Work out the finished part from the listing and answer in its coordinate system (mm). Coordinates: 2 decimals unless noted, no trailing zeros. Loops run counter-clockwise (first coordinate to the right, second up) from the corner with the lowest first, then second, coordinate; pieces in that order, holes last. Notation, with made-up numbers: (13, 13.25) -> (38, 13.25) arc R20 ccw to (38, 26.25) -> close; hole circle Ø7 at (71.5, 34). An arc over 180 degrees is marked (long way). Use a Markdown table: item, result.
from build123d import *

# Parameters (mm, degrees)
SKETCH1_R           = 30
SKETCH1_R_2         = 1.5
BOSS_EXTRUDE1_DEPTH = 8
SKETCH2_R           = 23.65
SKETCH2_R_2         = 7.62
CUT_EXTRUDE1_DEPTH  = 8
BOSS_EXTRUDE2_DEPTH = 8
CIRPATTERN1_COUNT   = 5


with BuildPart() as part:
    # Sketch1 → Boss-Extrude1 (new body)
    with BuildSketch(Plane(origin=(0, 0, 0), x_dir=(1, 0, 0), z_dir=(0, 1, 0))):
        with Locations(Location((0, 0, 0), (0, 0, 270))):
            Circle(SKETCH1_R)
        with Locations(Location((0, 0, 0), (0, 0, 270))):
            Circle(SKETCH1_R_2, mode=Mode.SUBTRACT)
    extrude(amount=BOSS_EXTRUDE1_DEPTH)

    # Sketch2 → Cut-Extrude1 (cut)
    with BuildSketch(Plane(origin=(0, 8, 0), x_dir=(1, 0, 0), z_dir=(0, 1, 0))):
        with Locations(Location((0, 0, 0), (0, 0, 270))):
            Circle(SKETCH2_R)
        with Locations(Location((0, 0, 0), (0, 0, 270))):
            Circle(SKETCH2_R_2, mode=Mode.SUBTRACT)
    extrude(amount=-CUT_EXTRUDE1_DEPTH, mode=Mode.SUBTRACT)


with BuildPart() as cut_extrude1_piece_1:
    # of the separate pieces the step leaves, piece 1, a body of its own (cut_extrude1_pieces)
    add(part.part.solids().sort_by_distance((0, 0, 30))[0])



with BuildPart() as cut_extrude1_piece_2:
    # of the separate pieces the step leaves, piece 2, a body of its own (cut_extrude1_pieces)
    add(part.part.solids().sort_by_distance((0, 0, 7.62))[0])


with BuildPart() as cut_extrude1_piece_1_1:
    add(cut_extrude1_piece_1.part)

    add(cut_extrude1_piece_2.part)  # Boss-Extrude2 merges Cut-Extrude1 piece 2
    # Sketch3 → Boss-Extrude2 (add)
    with BuildSketch(Plane(origin=(0, 8, 0), x_dir=(1, 0, 0), z_dir=(0, 1, 0))):
        with BuildLine():
            Line((-1.734503171, -8.366902694), (-1.734503171, -22.177406537))
            ThreePointArc((-1.734503171, -22.177406537), (-2.16892881, -23.133814131), (-3.175, -23.435909946))
            ThreePointArc((-3.175, -23.435909946), (0, -23.65), (3.175, -23.435909946))
            ThreePointArc((3.175, -23.435909946), (2.16892881, -23.133814131), (1.734503171, -22.177406537))
            Line((1.734503171, -22.177406537), (1.734503171, -8.366902694))
            ThreePointArc((1.734503171, -8.366902694), (1.965753269, -7.636219014), (2.575288432, -7.171630881))
            ThreePointArc((2.575288432, -7.171630881), (0, -7.62), (-2.575288432, -7.171630881))
            ThreePointArc((-2.575288432, -7.171630881), (-1.965753269, -7.636219014), (-1.734503171, -8.366902694))
        make_face()
    boss_extrude2 = extrude(amount=-BOSS_EXTRUDE2_DEPTH)

    # CirPattern1: Boss-Extrude2 ×5 about axis
    cirpattern1_axis = Axis((0, 0, 0), (0, 1, 0))
    for i in range(1, CIRPATTERN1_COUNT):
        add(boss_extrude2.rotate(cirpattern1_axis, i * 360 / CIRPATTERN1_COUNT))


solid = cut_extrude1_piece_1_1.part
Q1. Consider line 1 (X direction, y = 6.75, z = 0.5); line 2 (Z direction, x = -19.5, y = 1.25); line 3 (X direction, y = 6.5, z = -11.5). Determine where each line is inside the solid, lowest interval first. Write a range as [from, to].
Solved:
| item | result |
|---|---|
| line 1 | [-30, -23.64], [-7.88, -1.41], [1.41, 7.88], [23.64, 30] |
| line 2 | [-22.8, -13.38], [4.51, 8.16], [13.38, 22.8] |
| line 3 | [-27.71, -20.67], [-10.5, -6.21], [6.21, 10.5], [20.67, 27.71] |
Q2. Section C-C on y = 6.25 is taken. State how many separate pieces and enclosed holes the cut face has, and give its area (3 significant figures).
Solved:
| item | result |
|---|---|
| separate pieces | 1 |
| enclosed holes | 6 |
| area | 1,530 mm² |
Q3. Section D-D on z = 16.5 is taken. Determine the outline of the cut face in (x, y), and give its area (3 significant figures).
Solved:
| item | result |
|---|---|
| outline | (-25.05, 0) -> (-16.94, 0) -> (-16.94, 8) -> (-25.05, 8) -> close; (-1.73, 0) -> (1.73, 0) -> (1.73, 8) -> (-1.73, 8) -> close; (16.94, 0) -> (25.05, 0) -> (25.05, 8) -> (16.94, 8) -> close |
| area | 158 mm² |
Q4. Given pin 1 Ø1.5 at (x, y) = (5, 1.5) entering from -Z; pin 2 Ø2.5 at (x, z) = (0, 0) entering from -Y; pin 3 Ø1 at (x, y) = (-23, 4) entering from -Z; pin 4 Ø1.5 at (y, z) = (3, -4) entering from +X, each flat-ended and moving along its own axis, determine where each tip first touches the part or whether it passes through.
Solved:
| item | result |
|---|---|
| pin 1 | z = -29.7 |
| pin 2 | through |
| pin 3 | z = -19.84 |
| pin 4 | x = 29.82 |
Q5. Section B-B on z = -11.5 is taken. Determine the outline of the cut face in (x, y), and give its area (3 significant figures).
Solved:
| item | result |
|---|---|
| outline | (-27.71, 0) -> (-20.67, 0) -> (-20.67, 8) -> (-27.71, 8) -> close; (-10.5, 0) -> (-6.21, 0) -> (-6.21, 8) -> (-10.5, 8) -> close; (6.21, 0) -> (10.5, 0) -> (10.5, 8) -> (6.21, 8) -> close; (20.67, 0) -> (27.71, 0) -> (27.71, 8) -> (20.67, 8) -> close |
| area | 181 mm² |
Q6. Section A-A on x = 0 is taken. Determine the outline of the cut face in (y, z), and give its area (3 significant figures).
Solved:
| item | result |
|---|---|
| outline | (0, -30) -> (8, -30) -> (8, -23.65) -> (0, -23.65) -> close; (0, -7.62) -> (8, -7.62) -> (8, -1.5) -> (0, -1.5) -> close; (0, 1.5) -> (8, 1.5) -> (8, 30) -> (0, 30) -> close |
| area | 328 mm² |
